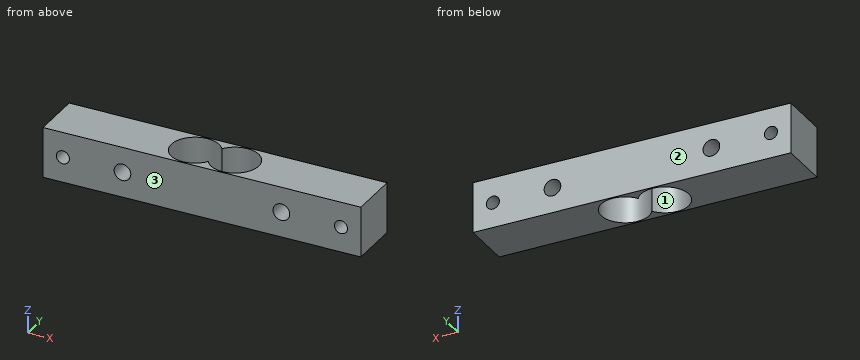
from build123d import *

# Parameters (mm, degrees)
SKETCH1_W                 = 80
SKETCH1_H                 = 12.7
BOSS_EXTRUDE1_DEPTH       = 6.35
SKETCH2_R                 = 6
CUT_EXTRUDE1_DEPTH        = 13.7
M4X0_7_TAPPED_HOLE2_D     = 3.3
M4X0_7_TAPPED_HOLE2_DEPTH = 12.7
M5X0_8_TAPPED_HOLE2_D     = 4.2
M5X0_8_TAPPED_HOLE2_DEPTH = 12.7


with BuildPart() as part:
    # Sketch1 → Boss-Extrude1 (new body, symmetric)
    with BuildSketch(Plane(origin=(0, 0, 0), x_dir=(1, 0, 0), z_dir=(0, 1, 0))):
        Rectangle(SKETCH1_W, SKETCH1_H)
    extrude(amount=BOSS_EXTRUDE1_DEPTH, both=True)

    # Sketch2 → Cut-Extrude1 (cut, through all)
    with BuildSketch(Plane.XY.offset(6.35)):
        with Locations((-5, 0)):
            Circle(SKETCH2_R)
        with Locations((5, 0)):
            Circle(SKETCH2_R)
    extrude(amount=-CUT_EXTRUDE1_DEPTH, mode=Mode.SUBTRACT)

    # M4x0.7 Tapped Hole2
    with Locations(Plane(origin=(0, 6.35, 0), x_dir=(1, 0, 0), z_dir=(0, 1, 0))):
        with Locations((-35, 0), (35, 0)):
            Hole(M4X0_7_TAPPED_HOLE2_D / 2, depth=M4X0_7_TAPPED_HOLE2_DEPTH)

    # M5x0.8 Tapped Hole2
    with Locations(Plane(origin=(0, 6.35, 0), x_dir=(1, 0, 0), z_dir=(0, 1, 0))):
        with Locations((20, 0), (-20, 0)):
            Hole(M5X0_8_TAPPED_HOLE2_D / 2, depth=M5X0_8_TAPPED_HOLE2_DEPTH)


solid = part.part
Input: part model. Units: mm. Frame: model coordinates. Face numbers are marked on the shaded views. Give positions to 0.01 mm unless a question says otherwise; leave off trailing zeros. Loops run counter-clockwise (first coordinate to the right, second up) from the corner with the lowest first, then second, coordinate; pieces in that order, holes last. Notation, with made-up numbers: (-40, 51.5) -> (-24, 51.5) arc R10 cw to (-24, 64.5) -> close; hole circle Ø3 at (61.5, -36.5). An arc over 180 degrees is marked (long way). Answer as a JSON object with one key per item and string values. Group by question number.
Item 1: Line query: probe 1 along Z at (x, y) = (35, 0.5); probe 2 along Y at (x, z) = (5, -1.5); probe 3 along X at (y, z) = (4.25, 4.25). Output: solid intervals per line, ascending.
Item 2: Cut plane A-A, the plane y = 0. Return the cut outline in (x, z), and give its area (3 significant figures).
Item 3: Cut plane D-D, the plane y = 4. Return the cut outline in (x, z).
Item 4: Cut plane C-C, the plane z = 0. Return the cut outline in (x, y), and give its area (3 significant figures).
Item 5: Pull-direction query (Y, two-part tool) for the marked faces 1, 2 and 3; classes: released by +Y, released by -Y, zero draft, split by the parting line, or undercut.
Item 6: Cut plane B-B, the plane x = 20. Return the cut outline in (y, z).
Checks:
{
 "1": {"probe 1": "z = -6.35 to -1.65, 1.65 to 6.35", "probe 2": "y = -6.35 to -6, 6 to 6.35", "probe 3": "x = -40 to -9.24, -0.76 to 0.76, 9.24 to 40"},
 "2": {"outline": "(-40, -6.35) -> (-11, -6.35) -> (-11, 6.35) -> (-40, 6.35) -> close; (11, -6.35) -> (40, -6.35) -> (40, 6.35) -> (11, 6.35) -> close; hole circle Ø3.3 at (-35, 0); hole circle Ø4.2 at (-20, 0); hole circle Ø4.2 at (20, 0); hole circle Ø3.3 at (35, 0)", "area": "692 mm²"},
 "3": {"outline": "(-40, -6.35) -> (-9.47, -6.35) -> (-9.47, 6.35) -> (-40, 6.35) -> close; (-0.53, -6.35) -> (0.53, -6.35) -> (0.53, 6.35) -> (-0.53, 6.35) -> close; (9.47, -6.35) -> (40, -6.35) -> (40, 6.35) -> (9.47, 6.35) -> close; hole circle Ø3.3 at (-35, 0); hole circle Ø4.2 at (-20, 0); hole circle Ø4.2 at (20, 0); hole circle Ø3.3 at (35, 0)"},
 "4": {"outline": "(-40, -6.35) -> (-36.65, -6.35) -> (-36.65, 6.35) -> (-40, 6.35) -> close; (-33.35, -6.35) -> (-22.1, -6.35) -> (-22.1, 6.35) -> (-33.35, 6.35) -> close; (-17.9, -6.35) -> (17.9, -6.35) -> (17.9, 6.35) -> (-17.9, 6.35) -> close; (22.1, -6.35) -> (33.35, -6.35) -> (33.35, 6.35) -> (22.1, 6.35) -> close; (36.65, -6.35) -> (40, -6.35) -> (40, 6.35) -> (36.65, 6.35) -> close; hole (0, -3.32) arc R6 ccw (long way) to (0, 3.32) arc R6 ccw (long way) to start", "area": "608 mm²"},
 "5": {"face 1": "undercut", "face 2": "released by +Y", "face 3": "released by -Y"},
 "6": {"outline": "(-6.35, -6.35) -> (6.35, -6.35) -> (6.35, -2.1) -> (-6.35, -2.1) -> close; (-6.35, 2.1) -> (6.35, 2.1) -> (6.35, 6.35) -> (-6.35, 6.35) -> close"}
}
